from build123d import *

# Parameters (mm, degrees)
BOSS_EXTRUDE1_DEPTH = 2
SKETCH5_W           = 2
SKETCH5_H           = 60
BOSS_EXTRUDE2_DEPTH = 55
SKETCH6_R           = 10
SKETCH6_R_2         = 1
CUT_EXTRUDE2_DEPTH  = 55
SKETCH8_R           = 2.585315043
CUT_EXTRUDE3_DEPTH  = 55
SKETCH4_W           = 30
SKETCH4_H           = 2
BOSS_EXTRUDE3_DEPTH = 20
CUT_EXTRUDE4_DEPTH  = 100


with BuildPart() as part:
    # Sketch2 → Boss-Extrude1 (new body)
    with BuildSketch(Plane.XY):
        with BuildLine():
            Line((-34, -30), (24, -30))
            ThreePointArc((24, -30), (31.071067812, -27.071067812), (34, -20))
            Line((34, -20), (34, 20))
            ThreePointArc((34, 20), (31.071067812, 27.071067812), (24, 30))
            Line((24, 30), (-34, 30))
            Line((-34, 30), (-34, -30))
        make_face()
    extrude(amount=BOSS_EXTRUDE1_DEPTH)

    # Sketch5 → Boss-Extrude2 (add)
    with BuildSketch(Plane.XY.offset(2)):
        with Locations((-33, 0)):
            Rectangle(SKETCH5_W, SKETCH5_H)
    extrude(amount=BOSS_EXTRUDE2_DEPTH)

    # Sketch6 → Cut-Extrude2 (cut)
    with BuildSketch(Plane.ZY.offset(34)):
        with Locations((28.5, 0)):
            Circle(SKETCH6_R)
        with Locations((40.277915604, 0)):
            Circle(SKETCH6_R_2)
        with Locations((36.828243992, -8.328243992)):
            Circle(SKETCH6_R_2)
        with Locations((28.5, -11.777915604)):
            Circle(SKETCH6_R_2)
        with Locations((20.171756008, -8.328243992)):
            Circle(SKETCH6_R_2)
        with Locations((16.722084396, 0)):
            Circle(SKETCH6_R_2)
        with Locations((20.171756008, 8.328243992)):
            Circle(SKETCH6_R_2)
        with Locations((28.5, 11.777915604)):
            Circle(SKETCH6_R_2)
        with Locations((36.828243992, 8.328243992)):
            Circle(SKETCH6_R_2)
        with BuildLine():
            Line((57, 30), (28.5, 30))
            ThreePointArc((28.5, 30), (48.739127681, 20.68967138), (57, 1.21e-07))
            Line((57, 1.21e-07), (57, 30))
        make_face()
        with BuildLine():
            Line((57, -30), (57, 1.21e-07))
            ThreePointArc((57, 1.21e-07), (48.739127764, -20.689671292), (28.5, -30))
            Line((28.5, -30), (57, -30))
        make_face()
    extrude(amount=-CUT_EXTRUDE2_DEPTH, mode=Mode.SUBTRACT)

    # Sketch8 → Cut-Extrude3 (cut)
    with BuildSketch(Plane.XY.offset(2)):
        with Locations((-21.5, 22.5)):
            Circle(SKETCH8_R)
        with BuildLine():
            Line((-11.5, 20), (-6.5, 20))
            ThreePointArc((-6.5, 20), (-4, 22.5), (-6.5, 25))
            Line((-6.5, 25), (-11.5, 25))
            ThreePointArc((-11.5, 25), (-14, 22.5), (-11.5, 20))
        make_face()
        with BuildLine():
            Line((8.5, 20), (13.5, 20))
            ThreePointArc((13.5, 20), (16, 22.5), (13.5, 25))
            Line((13.5, 25), (8.5, 25))
            ThreePointArc((8.5, 25), (6, 22.5), (8.5, 20))
        make_face()
        with Locations((21.5, 22.5)):
            Circle(SKETCH8_R)
        with BuildLine():
            Line((8.786451989, 16.481383401), (8.786451989, -14.819395159))
            ThreePointArc((8.786451989, -14.819395159), (11, -17.03294317), (13.213548011, -14.819395159))
            Line((13.213548011, -14.819395159), (13.213548011, 16.481383401))
            ThreePointArc((13.213548011, 16.481383401), (11, 18.694931413), (8.786451989, 16.481383401))
        make_face()
        with BuildLine():
            Line((-11.213548011, 16.481383401), (-11.213548011, -14.819395159))
            ThreePointArc((-11.213548011, -14.819395159), (-9, -17.03294317), (-6.786451989, -14.819395159))
            Line((-6.786451989, -14.819395159), (-6.786451989, 16.481383401))
            ThreePointArc((-6.786451989, 16.481383401), (-9, 18.694931413), (-11.213548011, 16.481383401))
        make_face()
        with Locations((-21.5, -22.5)):
            Circle(SKETCH8_R)
        with BuildLine():
            ThreePointArc((-6.5, -20), (-4, -22.5), (-6.5, -25))
            Line((-6.5, -25), (-11.5, -25))
            ThreePointArc((-11.5, -25), (-14, -22.5), (-11.5, -20))
            Line((-11.5, -20), (-6.5, -20))
        make_face()
        with BuildLine():
            ThreePointArc((13.5, -20), (16, -22.5), (13.5, -25))
            Line((13.5, -25), (8.5, -25))
            ThreePointArc((8.5, -25), (6, -22.5), (8.5, -20))
            Line((8.5, -20), (13.5, -20))
        make_face()
        with Locations((21.5, -22.5)):
            Circle(SKETCH8_R)
    extrude(amount=-CUT_EXTRUDE3_DEPTH, mode=Mode.SUBTRACT)

    # Sketch4 → Boss-Extrude3 (add)
    with BuildSketch(Plane.XY.offset(2)):
        with Locations((-19, -29)):
            Rectangle(SKETCH4_W, SKETCH4_H)
        with Locations((-19, 29)):
            Rectangle(SKETCH4_W, SKETCH4_H)
    extrude(amount=BOSS_EXTRUDE3_DEPTH)

    # Sketch10 → Cut-Extrude4 (cut)
    with BuildSketch(Plane.XZ.offset(30)):
        Polygon((-32, 22), (-4, 2), (-4, 22), align=None)
    extrude(amount=-CUT_EXTRUDE4_DEPTH, mode=Mode.SUBTRACT)


solid = part.part
The model under review builds one solid part; all positions refer to its coordinate system, in mm. A direction names the side the tool comes from. Coordinates: 2 decimals unless noted, no trailing zeros. Loops run counter-clockwise (first coordinate to the right, second up) from the corner with the lowest first, then second, coordinate; pieces in that order, holes last. Notation, with made-up numbers: (34.5, 70.5) -> (56.5, 70.5) arc R9 ccw to (56.5, 77.5) -> close; hole circle Ø2 at (19.25, 45.25). An arc over 180 degrees is marked (long way). Use a Markdown table: item, result. Add a question column.
1. Add section C-C on z = 24. Write out the cut boundary in (x, y).
2. Clearance check with flat-ended pins moving along their axes: pin 1 Ø12 at (y, z) = (19, 8.5) entering from +X; pin 2 Ø6 at (x, y) = (-21.5, 22.5) entering from +Z. State where each tip first meets the part, or that it passes through.
3. To check wall thickness, follow line 1 (Y direction, x = -32.45, z = 28.5); line 2 (Y direction, x = -30.5, z = 12); line 3 (X direction, y = 22, z = 18.5). State the ranges of each line that lie inside material, in increasing order.
4. Add section B-B on x = 21.5. Write out the cut boundary in (y, z), plus the area to 3 significant figures.
5. Machinability: for faces 1 (the face through (-32, 6, 17)), 2 (the face through (6, 22.6, 1)), 3 (the face through (-33.01, 3, 38.04)), which of the approach directions +Z, -Z, +X, -X, +Y, -Y give a long, thin tool a straight path to every point of the face, cutting with its end or side? Answer none if there is none.
6. Draft analysis for pull direction Y (two halves, no side actions). For faces 4 (the face through (-21.837, 25.063, 1.014)), 5 (the face through (0, 0, 0)), 6 (the face through (-20, -30, 7)), state which applies: pulls with the +Y half, pulls with the -Y half, needs draft (parallel to the pull), parting line crosses it, or undercut.
7. Add section D-D on y = -16. Write out the cut boundary in (x, z), plus the area to 3 significant figures.
8. Add section A-A on y = 0. Write out the cut boundary in (x, z), plus the area to 3 significant figures.
Returned:
| question | item | result |
|---|---|---|
| 1 | outline | (-34, -30) -> (-32, -30) -> (-32, -8.93) -> (-34, -8.93) -> close; (-34, 8.93) -> (-32, 8.93) -> (-32, 30) -> (-34, 30) -> close |
| 2 | pin 1 | stops at x = -32 |
| 2 | pin 2 | stops at z = 2 |
| 3 | line 1 | y = -30 to -12.78, -10.78 to -10, 10 to 10.78, 12.78 to 30 |
| 3 | line 2 | y = -30 to -28, 28 to 30 |
| 3 | line 3 | x = -34 to -32 |
| 4 | outline | (-30, 0) -> (-25.09, 0) -> (-25.09, 2) -> (-30, 2) -> close; (-19.91, 0) -> (19.91, 0) -> (19.91, 2) -> (-19.91, 2) -> close; (25.09, 0) -> (30, 0) -> (30, 2) -> (25.09, 2) -> close |
| 4 | area | 99.3 mm² |
| 5 | face 1 | +Z, +X |
| 5 | face 2 | +Z, -Z |
| 5 | face 3 | +X, -X |
| 6 | face 4 | undercut |
| 6 | face 5 | needs draft |
| 6 | face 6 | pulls with the -Y half |
| 7 | outline | (-34, 0) -> (-10.87, 0) -> (-10.87, 2) -> (-32, 2) -> (-32, 52.38) -> (-34, 52.38) -> close; (-7.13, 0) -> (9.13, 0) -> (9.13, 2) -> (-7.13, 2) -> close; (12.87, 0) -> (34, 0) -> (34, 2) -> (12.87, 2) -> close |
| 7 | area | 222 mm² |
| 8 | outline | (-34, 0) -> (-11.21, 0) -> (-11.21, 2) -> (-32, 2) -> (-32, 15.72) -> (-34, 15.72) -> close; (-34, 17.72) -> (-32, 17.72) -> (-32, 18.5) -> (-34, 18.5) -> close; (-34, 38.5) -> (-32, 38.5) -> (-32, 39.28) -> (-34, 39.28) -> close; (-34, 41.28) -> (-32, 41.28) -> (-32, 57) -> (-34, 57) -> close; (-6.79, 0) -> (8.79, 0) -> (8.79, 2) -> (-6.79, 2) -> close; (13.21, 0) -> (34, 0) -> (34, 2) -> (13.21, 2) -> close |
| 8 | area | 180 mm² |
